CAD build for the part. Positions are in the model's coordinates, mm. A direction names the side the tool comes from. Round coordinates to 2 decimals unless told otherwise and drop trailing zeros. Order: outer loops, then holes, each group sorted by start corner. A loop starts at its lowest first (then second) coordinate and runs counter-clockwise, first axis right, second up. Notation, with made-up numbers: M 68.25,35 L 119.25,35 A15 cw 119.25,51 Z; hole C -28.75,86.25 d10. An arc over 180 degrees is marked long. Put each result on its own line as item: value.
```python
from build123d import *

# Parameters (mm, degrees)
BOSS_EXTRUDE1_DEPTH = 5
SKETCH3_W           = 8
SKETCH3_H           = 4
BOSS_EXTRUDE2_DEPTH = 3
FILLET1_START       = -3.841593316
FILLET1_DEPTH       = 8
CUT_EXTRUDE1_START  = -10
CUT_EXTRUDE1_DEPTH  = 10


with BuildPart() as part:
    # Sketch1 → Boss-Extrude1 (new body)
    with BuildSketch(Plane(origin=(0, 0, 0), x_dir=(1, 0, 0), z_dir=(0, 1, 0))):
        with BuildLine():
            Line((-30, 0), (30, 0))
            ThreePointArc((30, 0), (0, 30), (-30, 0))
        make_face()
    extrude(amount=BOSS_EXTRUDE1_DEPTH)

    # Sketch3 → Boss-Extrude2 (add)
    with BuildSketch(Plane(origin=(0, 5, 0), x_dir=(1, 0, 0), z_dir=(0, 1, 0))):
        with Locations((0.158406684, 24.731666579)):
            Rectangle(SKETCH3_W, SKETCH3_H)
    extrude(amount=BOSS_EXTRUDE2_DEPTH)

    # Fillet1: read off the stored shape, not the designer's step
    # Fillet1 outline → Fillet1 (cut)
    with BuildSketch(Plane.YZ.offset(FILLET1_START)):
        with BuildLine():
            Line((8, -22.731666579), (5, -22.731666579))
            add(Edge.make_bspline(
                [(5, -22.731666579), (8, -23.506263249), (8, -26.604649926)],
                knots=[0, 0, 0, 1, 1, 1], degree=2, weights=[1, 0.057495957, 1]))
            Line((8, -26.604649926), (8, -22.731666579))
        make_face()
    extrude(amount=FILLET1_DEPTH, mode=Mode.SUBTRACT)

    # Sketch5 → Cut-Extrude1 (cut)
    with BuildSketch(Plane(origin=(0, 5, 0), x_dir=(1, 0, 0), z_dir=(0, 1, 0)).offset(CUT_EXTRUDE1_START)):
        with BuildLine():
            Line((-16.171904292, 0), (-16.171904292, 7))
            Line((-16.171904292, 7), (-29.171904292, 7))
            ThreePointArc((-29.171904292, 7), (-29.792256786, 3.524405712), (-30, 0))
            Line((-30, 0), (-16.171904292, 0))
        make_face()
        with BuildLine():
            Line((16.171904292, 7), (29.171904292, 7))
            ThreePointArc((29.171904292, 7), (29.792256786, 3.524405712), (30, 0))
            Line((30, 0), (16.171904292, 0))
            Line((16.171904292, 0), (16.171904292, 7))
        make_face()
    extrude(amount=CUT_EXTRUDE1_DEPTH, mode=Mode.SUBTRACT)


solid = part.part
```
Item 1: Band-saw the part on C-C on x = -12. Give the cut face in (y, z).
Answers below:
outline: M 0,-27.5 L 5,-27.5 L 5,0 L 0,0 Z
Item 2: Tool access for faces 1 (the flat face through (0, 6, -26.732)), 2 (the flat face through (-23, 2, -7)), 3 (the flat face through (16.172, 2, -3)), 4 (the flat face through (-3.842, 6, -25)): list every direction of +Z, -Z, +X, -X, +Y, -Y with a clear straight run to the whole face (end or side of a thin tool).
Answers below:
face 1: -Z, +X, -X, +Y
face 2: +Z, -X, +Y, -Y
face 3: +Z, +X, +Y, -Y
face 4: +Z, -Z, -X, +Y
Item 3: Band-saw the part on A-A on y = 1. Give the cut face in (x, z).
Answers below:
outline: M -29.17,-7 A30 ccw 29.17,-7 L 16.17,-7 L 16.17,0 L -16.17,0 L -16.17,-7 Z
Item 4: Probe line 1 along Y through (x, z) = (7, -20.5); line 2 along Z through (x, y) = (2.5, 1.75); line 3 along X through (y, z) = (0.75, -5.25). List the from-to ranges inside material, lowest first. Write a range as [from, to].
Answers below:
line 1: [0, 5]
line 2: [-29.9, 0]
line 3: [-16.17, 16.17]
Item 5: Pin check, flat tips, straight feed: P1, Ø3, axis at x = -20.5, z = -11.5, coming from the +Y side; P2, Ø2.5, axis at y = 6, z = -24.5, coming from the -X side; P3, Ø4, axis at x = -24.5, y = 3, coming from the +Z side. Stop position of each tip, or through.
Answers below:
P1: y = 5
P2: x = -18.33
P3: z = -7
Item 6: Band-saw the part on B-B on z = -5.25. Give the cut face in (x, y).
Answers below:
outline: M -16.17,0 L 16.17,0 L 16.17,5 L -16.17,5 Z
